Source: CAD feature listing. Evaluate the final solid. Frame: model axes, mm. Face numbers are marked on the shaded views. A direction names the side the tool comes from. Give positions to 0.01 mm unless a question says otherwise; leave off trailing zeros. Order: outer loops, then holes, each group sorted by start corner. A loop starts at its lowest first (then second) coordinate and runs counter-clockwise, first axis right, second up. Notation, with made-up numbers: (-16, 59) - (29, 59) arc R30 ccw to (29, 91) - close; hole circle Ø5 at (-28.75, 55). An arc over 180 degrees is marked (long way). Use CSV: the item, a comma, the result in double quotes.
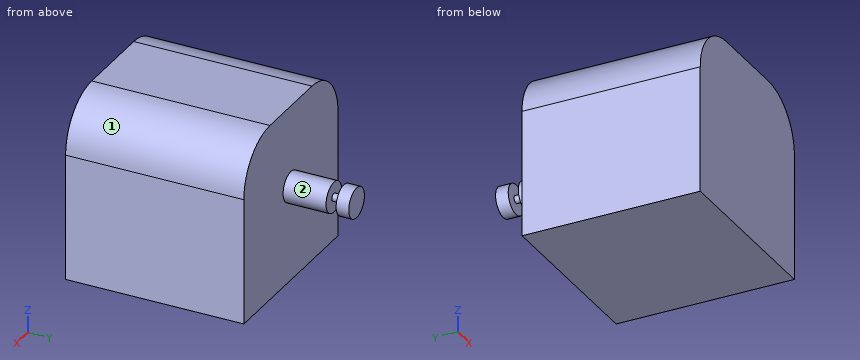
Autodesk Inventor part; units mm, degrees
ref_plane "YZ Plane" through (0, 0, 0) normal (1, 0, 0) x (0, 1, 0)
ref_plane "XZ Plane" through (0, 0, 0) normal (0, 1, 0) x (-1, 0, 0)
ref_plane "XY Plane" through (0, 0, 0) normal (0, 0, 1) x (1, 0, 0)
ref_plane "Plano de trabajo1" through (-56.2353, 9.9981, -187.965) normal (0, 0, 1) x (1, 0, 0)
sketch "Boceto1" plane through (-56.2353, 9.9981, -187.965) normal (0, 0, 1) x (1, 0, 0)
  line L0 (-114.1422, 169.9991) -> (-475.1878, 169.9991)
  line L1 (-475.1878, 169.9991) -> (-475.1878, -182.9514)
  line L2 (-475.1878, -182.9514) -> (-114.1422, -182.9514)
  line L3 (-114.1422, -182.9514) -> (-114.1422, 169.9991)
  point P0 (56.2353, -9.9981)
extrude "Extrusión1" add sketch "Boceto1" along normal blind 350
fillet "Empalme1" radius 100 2 edges at (-531.4231, 3.522, 162.035) (-170.3775, 3.522, 162.035)
sketch "Boceto2" plane through (-531.4231, 179.9972, -187.965) normal (0, 1, 0) x (1, 0, 0)
  circle A0 centre (180.5228, -187.965) radius 30
  point P0 (531.4231, -187.965)
  dimension "d3" = 60
extrude "Extrusión2" add sketch "Boceto2" along normal blind 85
sketch "Boceto5" plane through (-350.9003, 264.9972, 0) normal (0, 1, 0) x (1, 0, 0)
  circle A0 centre (0, 0) radius 7.5
  point P0 (350.9003, 0)
  dimension "d18" = 15
extrude "Extrusión5" add sketch "Boceto5" along normal blind 20
sketch "Boceto6" plane through (-350.9003, 284.9972, 0) normal (0, 1, 0) x (1, 0, 0)
  circle A0 centre (0, 0) radius 7.5
  circle A1 centre (0, 0) radius 30
  point P0 (350.9003, 0)
  dimension "d21" = 60
extrude "Extrusión6" add sketch "Boceto6" along normal blind 25 contours A0 | A1
Item 1: Material intervals for line 1 (Y direction, x = -459, z = -8); line 2 (X direction, y = 95.5, z = 63.5); line 3 (Z direction, x = -222, y = 20.5) (3 decimals), sorted ascending. Write a range as from..to.
Filled in:
line 1,"y = -172.95..180"
line 2,"x = -531.41..-170.39"
line 3,"z = -187.965..149.554"
Item 2: Set-up query: the marked faces 1 and 2. Return all of +Z, -Z, +X, -X, +Y, -Y with unobstructed straight access to the full face (end or side cutting, diameter ignored); none if empty.
Filled in:
face 1,"+Z, +X, +Y, -Y"
face 2,"+Y"
Item 3: First-contact query: pin 1 (3 mm diameter, centred on x = -255.5, z = 81.5, fed in from +Y); pin 2 (10 mm diameter, centred on x = -208, y = -119, fed in from +Z); pin 3 (12 mm diameter, centred on x = -264, y = 99.5, fed in from +Z). Flat tips, straight axial feed; report the tip coordinate or a pass-through.
Filled in:
pin 1,"stops at y = 180"
pin 2,"stops at z = 143.94"
pin 3,"stops at z = 162.03"
Item 4: Section C-C on y = -14.5. Return the cut outline in (x, z) (1 decimal), then the cut area to 3 significant figures.
Filled in:
outline,"(-531.4, -188) - (-170.4, -188) - (-170.4, 62) arc R100 ccw to (-270.4, 162) - (-431.4, 162) arc R100 ccw to (-531.4, 62) - close"
area,"122,000 mm2"
Item 5: Section A-A on z = 0. Return the cut outline in (x, y), then the cut area to 3 significant figures.
Filled in:
outline,"(-531.42, -172.95) - (-170.38, -172.95) - (-170.38, 180) - (-320.9, 180) - (-320.9, 265) - (-343.4, 265) - (-343.4, 285) - (-320.9, 285) - (-320.9, 310) - (-380.9, 310) - (-380.9, 285) - (-358.4, 285) - (-358.4, 265) - (-380.9, 265) - (-380.9, 180) - (-531.42, 180) - close"
area,"134,000 mm2"
Item 6: Section B-B on x = -302.5. Return the cut outline in (y, z) (3 decimals).
Filled in:
outline,"(-172.953, -187.965) - (179.997, -187.965) - (179.997, 162.035) - (-172.953, 162.035) - close"
Item 7: Section D-D on z = -77. Return the cut outline in (x, y).
Filled in:
outline,"(-531.42, -172.95) - (-170.38, -172.95) - (-170.38, 180) - (-531.42, 180) - close"
